Autodesk Inventor part; units mm, degrees
ref_plane "YZ Plane" through (0, 0, 0) normal (1, 0, 0) x (0, 1, 0)
ref_plane "XZ Plane" through (0, 0, 0) normal (0, 1, 0) x (-1, 0, 0)
ref_plane "XY Plane" through (0, 0, 0) normal (0, 0, 1) x (1, 0, 0)
sketch "スケッチ1" plane through (0, 0, 0) normal (0, 0, 1) x (1, 0, 0)
  circle A0 centre (0, 0) radius 10
  line L0 (22.5, 10) -> (-22.5, 10) construction
  line L1 (-22.5, 10) -> (-22.5, -10) construction
  line L2 (-22.5, -10) -> (22.5, -10) construction
  line L3 (22.5, -10) -> (22.5, 10) construction
  line L4 (22.5, 10) -> (-22.5, -10) construction
  line L5 (-22.5, 10) -> (22.5, -10) construction
  circle A1 centre (-22.5, 10) radius 1.25
  circle A2 centre (-22.5, -10) radius 1.25
  circle A3 centre (22.5, 10) radius 1.25
  circle A4 centre (22.5, -10) radius 1.25
  circle A5 centre (0, 0) radius 25 construction
  line L6 (20, 20) -> (-20, 20) construction
  line L7 (-20, 20) -> (-20, -20) construction
  line L8 (-20, -20) -> (20, -20) construction
  line L9 (20, -20) -> (20, 20) construction
  line L10 (20, 20) -> (-20, -20) construction
  line L11 (-20, 20) -> (20, -20) construction
  circle A6 centre (-20, 20) radius 1.25
  circle A7 centre (20, 20) radius 1.25
  circle A8 centre (20, -20) radius 1.25
  circle A9 centre (-20, -20) radius 1.25
  arc A10 (-20, 24) -> (-23.9564, 20.5891) centre (-20, 20) ccw
  arc A11 (-25.4673, 10.4418) -> (-25.5, 10) centre (-22.5, 10) ccw
  arc A12 (-25.5, -10) -> (-25.4673, -10.4418) centre (-22.5, -10) ccw
  arc A13 (-23.9564, -20.5891) -> (-20, -24) centre (-20, -20) ccw
  arc A14 (20, -24) -> (23.9564, -20.5891) centre (20, -20) ccw
  arc A15 (25.4673, -10.4418) -> (25.5, -10) centre (22.5, -10) ccw
  arc A16 (25.5, 10) -> (25.4673, 10.4418) centre (22.5, 10) ccw
  arc A17 (23.9564, 20.5891) -> (20, 24) centre (20, 20) ccw
  line L12 (-23.9564, 20.5891) -> (-25.4673, 10.4418)
  line L13 (-20, 24) -> (20, 24)
  line L14 (23.9564, 20.5891) -> (25.4673, 10.4418)
  line L15 (25.5, 10) -> (25.5, -10)
  line L16 (25.4673, -10.4418) -> (23.9564, -20.5891)
  line L17 (20, -24) -> (-20, -24)
  line L18 (-23.9564, -20.5891) -> (-25.4673, -10.4418)
  line L19 (-25.5, 10) -> (-25.5, -10)
  dimension "d0" = 20
  dimension "d1" = 45
  dimension "d2" = 20
  dimension "d3" = 2.5
  dimension "d4" = 2.5
  dimension "d5" = 2.5
  dimension "d6" = 2.5
  dimension "d7" = 50
  dimension "d8" = 40
  dimension "d9" = 40
  dimension "d10" = 2.5
  dimension "d11" = 2.5
  dimension "d12" = 2.5
  dimension "d13" = 2.5
  dimension "d14" = 4
  dimension "d15" = 4
  dimension "d16" = 3
  dimension "d17" = 3
  dimension "d18" = 4
  dimension "d19" = 4
  dimension "d20" = 3
  dimension "d21" = 3
extrude "押し出し1" add sketch "スケッチ1" along normal blind 3
properties part number "関節3_775側_プーリ側板" material "アルミニウム 6061"
Part model, mm, in its own coordinate system. Give positions to 0.01 mm unless a question says otherwise; leave off trailing zeros. Write each loop counter-clockwise with the first axis right and the second up, starting at its lowest first coordinate (ties: lowest second). Pieces come first, ordered by that corner, then holes.
1) Two-plate mould, pull along Y, no slides. Class faces 1 (the face through (21.155, 20.479, 1.479)), 2 (the face through (0, 11, 3)), 3 (the face through (0, -24, 1)): released by +Y, released by -Y, zero draft, split by the parting line, or undercut.
Resolved:
face 1: undercut
face 2: zero draft
face 3: released by -Y
2) Probe L1, parallel to Y at x = 20, z = 1.9; L2, parallel to Y at x = 0, z = 0.85; L3, parallel to X at y = -11, z = 2.35. List the from-to ranges inside material, lowest first.
Resolved:
L1: y = -24 to -21.25, -18.75 to 18.75, 21.25 to 24
L2: y = -24 to -10, 10 to 24
L3: x = -25.38 to -23.25, -21.75 to 21.75, 23.25 to 25.38
3) Cut at A-A on y = 0. Write the cut outline in (x, z).
Resolved:
outline: (-25.5, 0) - (-10, 0) - (-10, 3) - (-25.5, 3) - close; (10, 0) - (25.5, 0) - (25.5, 3) - (10, 3) - close
4) Cut at C-C on x = -22.5. Write the cut outline in (y, z).
Resolved:
outline: (-23.12, 0) - (-11.25, 0) - (-11.25, 3) - (-23.12, 3) - close; (-8.75, 0) - (8.75, 0) - (8.75, 3) - (-8.75, 3) - close; (11.25, 0) - (23.12, 0) - (23.12, 3) - (11.25, 3) - close
5) Cut at D-D on y = -20. Write the cut outline in (x, z), then the cut area to 3 significant figures.
Resolved:
outline: (-24.04, 0) - (-21.25, 0) - (-21.25, 3) - (-24.04, 3) - close; (-18.75, 0) - (18.75, 0) - (18.75, 3) - (-18.75, 3) - close; (21.25, 0) - (24.04, 0) - (24.04, 3) - (21.25, 3) - close
area: 129 mm2
6) Cut at B-B on z = 1.55. State how many separate pieces and enclosed holes the cut face has, then the cut area to 3 significant figures.
Resolved:
separate pieces: 1
enclosed holes: 9
area: 2,030 mm2
